from build123d import *

# Parameters (mm, degrees)
F0_R     = 42.041892
F1_DEPTH = 63.5
F2_DEPTH = 12.7
F4_DEPTH = 6.35


with BuildPart() as f1:
    # F0 (on Top) → F1 (new body)
    with BuildSketch(Plane.XY):
        with BuildLine():
            ThreePointArc((52.548027, -53.411115), (108.062324, -48.95714), (134.611778, 0))
            ThreePointArc((134.611778, 0), (108.062324, 48.95714), (52.548027, 53.411115))
            ThreePointArc((52.548027, 53.411115), (17.785453, 0), (52.548027, -53.411115))
        make_face()
        with Locations((76.198615, 0)):
            Circle(F0_R, mode=Mode.SUBTRACT)
    extrude(amount=F1_DEPTH)

    # F0 (on Top) → F2 (join)
    with BuildSketch(Plane.XY):
        with BuildLine():
            ThreePointArc((52.548027, -53.411115), (17.785453, 0), (52.548027, 53.411115))
            Line((52.548027, 53.411115), (-52.548027, 53.411115))
            Line((-52.548027, 53.411115), (-52.548027, -53.411115))
            Line((-52.548027, -53.411115), (52.548027, -53.411115))
        make_face()
    extrude(amount=F2_DEPTH)

    # F3 (on Front) → F4 (join, symmetric)
    with BuildSketch(Plane.XZ):
        Polygon((17.915584, 12.179299), (17.915584, 55.029098), (-38.820458, 12.179299), align=None)
    extrude(amount=F4_DEPTH, both=True)


solid = f1.part
Build history of the part. All positions in model axes, mm. A direction names the side the tool comes from. Round coordinates to 2 decimals unless told otherwise and drop trailing zeros. Write each loop counter-clockwise with the first axis right and the second up, starting at its lowest first coordinate (ties: lowest second). Pieces come first, ordered by that corner, then holes. Notation, with made-up numbers: M 79.25,31 L 117.25,31 A27 cw 117.25,64 Z; hole C 28,-37.5 d6. An arc over 180 degrees is marked long. Answer as a JSON object with one key per item and string values. Group by question number.
(1) Cut at D-D (y = -47). Give the cut face in (x, z).
(2) Cut at B-B (x = 66). Give the cut face in (y, z), and give its area (3 significant figures).
(3) Which spindle directions (+Z, -Z, +X, -X, +Y, -Y) get a long thin tool onto all of the face, cutting with end or side? Do faces 1 (the flat face through (1, 53.411, 6)), 2 (the flat face through (2, -6.35, 25)), 3 (the flat face through (-52.548, 1, 6)). Say none if no direction does.
(4) Drill centre lines: L1, parallel to Z at x = -25.5, y = 42.5; L2, parallel to X at y = 37, z = 8.5; L3, parallel to X at y = -35.5, z = 60.5. Where is each one in solid material? Low to high.
(5) Cut at A-A (y = -24). Give the cut face in (x, z), and give its area (3 significant figures).
(6) Cut at C-C (z = 40). Give the cut face in (x, y), and give its area (3 significant figures).
(7) Flat gauge pins, fed straight in: pin 1 (1.5 mm diameter, centred on x = 47, z = 40, fed in from +Y); pin 2 (12 mm diameter, centred on y = -4, z = 13, fed in from +X); pin 3 (12.5 mm diameter, centred on x = -6, z = 23.5, fed in from +Y); pin 4 (4 mm diameter, centred on x = -1, z = 9.5, fed in from -Y). Where does each tip first touch, or does it go through?
(8) Mould opens along Y. For faces 4 (the flat face through (62, 40, 63.5)), 5 (the flat face through (2, 6.35, 25)), 6 (the cylindrical face through (98.8, 35.45, 31.31)), 7 (the flat face through (-1, -53.411, 6)) say: pulls with the +Y half, pulls with the -Y half, needs draft (parallel to the pull), parting line crosses it, or undercut.
Responses:
{
 "1": {"outline": "M -52.55,0 L 110.88,0 L 110.88,63.5 L 41.51,63.5 L 41.51,12.7 L -52.55,12.7 Z"},
 "2": {"outline": "M -57.52,0 L -40.79,0 L -40.79,63.5 L -57.52,63.5 Z; M 40.79,0 L 57.52,0 L 57.52,63.5 L 40.79,63.5 Z", "area": "2,120 mm2"},
 "3": {"face 1": "+Z, -Z, -X, +Y", "face 2": "+Z, -X, -Y", "face 3": "+Z, -Z, -X, +Y, -Y"},
 "4": {"L1": "z = 0 to 12.7", "L2": "x = -52.55 to 56.24, 96.16 to 121.4", "L3": "x = 29.81 to 53.68, 98.72 to 122.59"},
 "5": {"outline": "M -52.55,0 L 41.68,0 L 41.68,63.5 L 22.94,63.5 L 22.94,12.7 L -52.55,12.7 Z; M 110.72,0 L 129.45,0 L 129.45,63.5 L 110.72,63.5 Z", "area": "3,340 mm2"},
 "6": {"outline": "M -1.98,-6.35 L 17.92,-6.35 L 17.92,-3.9 A58.41 ccw 52.55,-53.41 A58.41 ccw 134.61,0 A58.41 ccw 52.55,53.41 A58.41 ccw 17.92,3.9 L 17.92,6.35 L -1.98,6.35 Z; hole C 76.2,0 d84.08", "area": "5,420 mm2"},
 "7": {"pin 1": "stops at y = 51.02", "pin 2": "stops at x = 134.61", "pin 3": "stops at y = 6.35", "pin 4": "stops at y = -53.41"},
 "8": {"face 4": "needs draft", "face 5": "pulls with the +Y half", "face 6": "undercut", "face 7": "pulls with the -Y half"}
}
